from build123d import *

# Parameters (mm, degrees)
F0_W     = 410
F0_H     = 100
F0_R     = 3.5
F1_DEPTH = 5


with BuildPart() as f1:
    # F0 (on Right) → F1 (new body)
    with BuildSketch(Plane.YZ):
        with Locations((0, 50)):
            Rectangle(F0_W, F0_H)
        with Locations((-160, 7)):
            Circle(F0_R, mode=Mode.SUBTRACT)
        with Locations((160, 7)):
            Circle(F0_R, mode=Mode.SUBTRACT)
        with Locations((-160, 55)):
            Circle(F0_R, mode=Mode.SUBTRACT)
        with Locations((160, 55)):
            Circle(F0_R, mode=Mode.SUBTRACT)
    extrude(amount=F1_DEPTH)


solid = f1.part
Work out the finished part from the listing and answer in its coordinate system (mm). Coordinates: 2 decimals unless noted, no trailing zeros. Write each loop counter-clockwise with the first axis right and the second up, starting at its lowest first coordinate (ties: lowest second). Pieces come first, ordered by that corner, then holes. Notation, with made-up numbers: M 69,38.25 L 125,38.25 A17 ccw 125,67.25 Z; hole C -16,15.25 d8. An arc over 180 degrees is marked long. Answer as CSV lines item,"result". Start each with the question number.
Item 1: Consider L1, parallel to Z at x = 2.45, y = 160. Determine where the line is inside the solid, lowest interval first.
Item 2: Section B-B on z = 7 is taken. Write down the section's boundary in (x, y), and give its area (3 significant figures).
Item 3: Section A-A on y = -160 is taken. Write down the section's boundary in (x, z), and give its area (3 significant figures).
Item 4: Determine the mould class of faces 1 (the face through (5, -3, 51)), 2 (the face through (2.46, -156.66, 8.05)) for opening direction Y: released by +Y, released by -Y, zero draft, split by the parting line, or undercut.
Item 5: Flat-ended cylindrical pins translate along their axes: P1, Ø8, axis at y = -160, z = 55, coming from the +X side; P2, Ø6.5, axis at y = 160, z = 7, coming from the -X side. Find the tip coordinate at first contact, or state that the pin passes through.
Checks:
1,L1,"z = 0 to 3.5, 10.5 to 51.5, 58.5 to 100"
2,outline,"M 0,-205 L 5,-205 L 5,-163.5 L 0,-163.5 Z; M 0,-156.5 L 5,-156.5 L 5,156.5 L 0,156.5 Z; M 0,163.5 L 5,163.5 L 5,205 L 0,205 Z"
2,area,"1,980 mm²"
3,outline,"M 0,0 L 5,0 L 5,3.5 L 0,3.5 Z; M 0,10.5 L 5,10.5 L 5,51.5 L 0,51.5 Z; M 0,58.5 L 5,58.5 L 5,100 L 0,100 Z"
3,area,"430 mm²"
4,face 1,"zero draft"
4,face 2,"undercut"
5,P1,"stops at x = 5"
5,P2,"passes through"
